Could you check a few things on this model? Use its own coordinates, in mm. Coordinates: 2 decimals unless noted, no trailing zeros. Write each loop counter-clockwise with the first axis right and the second up, starting at its lowest first coordinate (ties: lowest second). Pieces come first, ordered by that corner, then holes. Notation, with made-up numbers: (25, 1.5) - (62, 1.5) arc R24 cw to (62, 27.5) - close; hole circle Ø11 at (-10.5, 33). An arc over 180 degrees is marked (long way). Answer as a JSON object with one key per item and string values. Group by question number.
1) If we section it at D-D (x = -70): State how many separate pieces and enclosed holes the cut face has, plus the area to 3 significant figures.
2) Please list where these lines run through material, in increasing order: line 1 along Y through (x, z) = (-82, 25); line 2 along Z through (x, y) = (-78.5, 0); line 3 along Y through (x, z) = (-82.5, 12).
3) Will this pin go through, and if not, where does the flat tip stop? pin 1 Ø15 at (x, y) = (-62.73, -0.09) entering from -Z.
4) We'd pull the mould along Y, two halves only. Please class faces 1 (the cylindrical face through (-44.54, 8.06, 37.65)), 2 (the flat face through (-87.733, -12, 14)), 3 (the flat face through (-74.2, 24.913, 13.5)): released by +Y, released by -Y, zero draft, split by the parting line, or undercut.
5) If we section it at C-C (y = -20): Write out the boundary of the cut face in (x, z).
6) If we section it at A-A (z = 25): Write out the boundary of the cut face in (x, y), plus the area to 3 significant figures.
7) If we section it at B-B (x = -41.5): Write out the boundary of the cut face in (y, z), plus the area to 3 significant figures.
```python
from build123d import *

# Parameters (mm, degrees)
F0_W     = 50
F0_H     = 50
F1_DEPTH = 50
F2_R     = 15
F3_DEPTH = 50.001
F4_R     = 15
F5_DEPTH = 50.001
F6_R     = 12.5
F7_DEPTH = 50.001
F8_SIZE  = 1


with BuildPart() as f1:
    # F0 (on Top) → F1 (new body)
    with BuildSketch(Plane.XY):
        with Locations((-62.7328101546, -0.0872552718)):
            Rectangle(F0_W, F0_H)
    extrude(amount=F1_DEPTH)

    # F2 (on face) → F3 (cut, through all)
    with BuildSketch(Plane.XZ.offset(25.0872552718)):
        with Locations((-62.7328101546, 25)):
            Circle(F2_R)
    extrude(amount=-F3_DEPTH, mode=Mode.SUBTRACT)

    # F4 (on face) → F5 (cut, through all)
    with BuildSketch(Plane.YZ.offset(-37.7328101546)):
        with Locations((0, 25)):
            Circle(F4_R)
    extrude(amount=-F5_DEPTH, mode=Mode.SUBTRACT)

    # F6 (on face) → F7 (cut, through all)
    with BuildSketch(Plane.XY.offset(50)):
        with Locations((-62.7328101546, -0.0872552718)):
            Circle(F6_R)
    extrude(amount=-F7_DEPTH, mode=Mode.SUBTRACT)

    # F8
    f8_edges = [f1.edges().sort_by_distance(p)[0] for p in [
        (-77.73281, -25.087255, 25),
        (-37.73281, -15, 25),
        (-75.23281, -0.087255, 50),
        (-77.73281, 24.912745, 25),
        (-75.23281, -0.087255, 0),
        (-87.73281, -15, 25),
    ]]
    chamfer(f8_edges, length=F8_SIZE)


solid = f1.part
```
Here are the results:
{
 "1": {"separate pieces": "4", "enclosed holes": "0", "area": "700 mm²"},
 "2": {"line 1": "y = -25.09 to -15, 15 to 24.91", "line 2": "z = 0 to 10, 40 to 50", "line 3": "y = -25.09 to -7.48, 7.48 to 24.91"},
 "3": {"pin 1": "passes through"},
 "4": {"face 1": "undercut", "face 2": "zero draft", "face 3": "released by +Y"},
 "5": {"outline": "(-87.73, 0) - (-37.73, 0) - (-37.73, 50) - (-87.73, 50) - close; hole circle Ø30 at (-62.73, 25)"},
 "6": {"outline": "(-87.73, -25.09) - (-78.73, -25.09) - (-77.73, -24.09) - (-77.73, -15) - (-86.73, -15) - (-87.73, -16) - close; (-87.73, 16) - (-86.73, 15) - (-77.73, 15) - (-77.73, 23.91) - (-78.73, 24.91) - (-87.73, 24.91) - close; (-47.73, -24.09) - (-46.73, -25.09) - (-37.73, -25.09) - (-37.73, -16) - (-38.73, -15) - (-47.73, -15) - close; (-47.73, 15) - (-38.73, 15) - (-37.73, 16) - (-37.73, 24.91) - (-46.73, 24.91) - (-47.73, 23.91) - close", "area": "396 mm²"},
 "7": {"outline": "(-25.09, 0) - (24.91, 0) - (24.91, 50) - (-25.09, 50) - close; hole circle Ø30 at (0, 25)", "area": "1,790 mm²"}
}
